Build history of the part. All positions in model axes, mm. Face numbers are marked on the shaded views. A direction names the side the tool comes from. Round coordinates to 2 decimals unless told otherwise and drop trailing zeros. Order: outer loops, then holes, each group sorted by start corner. A loop starts at its lowest first (then second) coordinate and runs counter-clockwise, first axis right, second up. Notation, with made-up numbers: M -28,19.5 L 5,19.5 A14 cw 5,36.5 Z; hole C 71,-7 d1. An arc over 180 degrees is marked long. One line per question, with ' | ' between items. Start each with the question number.
from build123d import *

# Parameters (mm, degrees)
SKETCH1_R           = 2.5
BOSS_EXTRUDE1_DEPTH = 10
SKETCH2_W           = 4
SKETCH2_H           = 61.321004691
CUT_EXTRUDE1_DEPTH  = 3
FILLET1_R           = 5
CHAMFER2_SIZE       = 4
CHAMFER3_SIZE       = 4
SKETCH3_R           = 2.5
CUT_EXTRUDE2_DEPTH  = 10


with BuildPart() as part:
    # Sketch1 → Boss-Extrude1 (new body)
    with BuildSketch(Plane(origin=(0, 0, 0), x_dir=(1, 0, 0), z_dir=(0, 1, 0))):
        Polygon((0, -25), (0, 25), (15, 25), (15, -8), (20, -16), (24.76, -16), (24.76, -22.47), (30.26, -22.47), (30.26, -18), (35, -18), (120, -18), (120, -33), (5, -33), align=None)
        with Locations(Location((5, 20, 0), (0, 0, 270))):
            Circle(SKETCH1_R, mode=Mode.SUBTRACT)
        with Locations(Location((5, -20, 0), (0, 0, 270))):
            Circle(SKETCH1_R, mode=Mode.SUBTRACT)
    extrude(amount=BOSS_EXTRUDE1_DEPTH)

    # Sketch2 → Cut-Extrude1 (cut)
    with BuildSketch(Plane(origin=(0, 10, 0), x_dir=(1, 0, 0), z_dir=(0, 1, 0))):
        with Locations((12, -5.660502345)):
            Rectangle(SKETCH2_W, SKETCH2_H)
    extrude(amount=-CUT_EXTRUDE1_DEPTH, mode=Mode.SUBTRACT)

    # Fillet1
    fillet1_edges = [part.edges().sort_by_distance(p)[0] for p in [
        (120, 5, 33),
        (120, 5, 18),
        (0, 5, -25),
        (15, 5, -25),
    ]]
    fillet(fillet1_edges, radius=FILLET1_R)

    # Chamfer2
    # the kernel refuses this chamfer: 4 mm, written as the material it takes off along each edge
    with BuildSketch(Plane(origin=(115, 10, 33), x_dir=(0, -0.9996219169112968, 0.02749587661058563), z_dir=(-1, 0, 0))) as chamfer2_piece_1:
        Polygon((CHAMFER2_SIZE * 0.999621916911, -CHAMFER2_SIZE * 0.0274958766106), (-CHAMFER2_SIZE * 0.0274958766106, -CHAMFER2_SIZE * 0.999621916911), (0, 0), align=None)
    extrude(amount=111.286731952, mode=Mode.SUBTRACT)
    with BuildSketch(Plane(origin=(20.286731952, 10, 33), x_dir=(0, 0.027495876610586487, -0.9996219169112968), z_dir=(-1, 0, 0))) as chamfer2_piece_2:
        Polygon((CHAMFER2_SIZE * 0.999621916911, CHAMFER2_SIZE * 0.0274958766106), (-CHAMFER2_SIZE * 0.0274958766106, CHAMFER2_SIZE * 0.999621916911), (0, 0), align=None)
    extrude(amount=25.573463904, mode=Mode.SUBTRACT)
    with BuildSketch(Plane(origin=(115, 10, 28), x_dir=(0, 0, 1), z_dir=(-1, 0, 0))) as chamfer2_piece_3:
        Polygon((5, -CHAMFER2_SIZE), (5 - CHAMFER2_SIZE, 0), (5, 0), align=None)
    revolve(axis=Axis((115, 10, 28), (0, 1, 0)), revolution_arc=90, mode=Mode.SUBTRACT)
    with BuildSketch(Plane(origin=(120, 10, 23), x_dir=(0.02749587661058563, -0.9996219169112968, 0), z_dir=(0, 0, 1))) as chamfer2_piece_4:
        Polygon((CHAMFER2_SIZE * 0.999621916911, -CHAMFER2_SIZE * 0.0274958766106), (-CHAMFER2_SIZE * 0.0274958766106, -CHAMFER2_SIZE * 0.999621916911), (0, 0), align=None)
    extrude(amount=5, mode=Mode.SUBTRACT)
    with BuildSketch(Plane(origin=(115, 10, 23), x_dir=(0, 0, -1), z_dir=(-1, 0, 0))) as chamfer2_piece_5:
        Polygon((5, CHAMFER2_SIZE), (5 - CHAMFER2_SIZE, 0), (5, 0), align=None)
    revolve(axis=Axis((115, 10, 23), (0, -1, 0)), revolution_arc=90, mode=Mode.SUBTRACT)
    with BuildSketch(Plane(origin=(30.26, 10, 18), x_dir=(0, -0.9996219169112968, -0.027495876610586494), z_dir=(1, 0, 0))) as chamfer2_piece_6:
        Polygon((CHAMFER2_SIZE * 0.999621916911, -CHAMFER2_SIZE * 0.0274958766106), (-CHAMFER2_SIZE * 0.0274958766106, -CHAMFER2_SIZE * 0.999621916911), (0, 0), align=None)
    extrude(amount=84.74, mode=Mode.SUBTRACT)

    # Chamfer3
    chamfer3_edges = [part.edges().sort_by_distance(p)[0] for p in [
        (22.38, 10, 16),
        (17.5, 10, 12),
    ]]
    chamfer(chamfer3_edges, length=CHAMFER3_SIZE)

    # Sketch3 → Cut-Extrude2 (cut)
    with BuildSketch(Plane(origin=(0, 10, 0), x_dir=(1, 0, 0), z_dir=(0, 1, 0))):
        with Locations(Location((27.5, -27, 0), (0, 0, 270))):
            Circle(SKETCH3_R)
    extrude(amount=-CUT_EXTRUDE2_DEPTH, mode=Mode.SUBTRACT)


solid = part.part
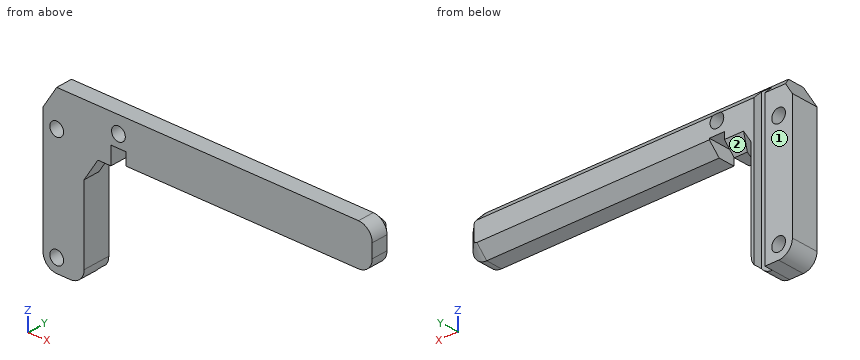
Item 1: Cut at B-B on x = 54. Write the cut outline in (y, z), then the cut area to 3 significant figures.
Item 2: Tool access for the marked faces 1 and 2: list every direction of +Z, -Z, +X, -X, +Y, -Y with a clear straight run to the whole face (end or side of a thin tool).
Item 3: Flat gauge pins, fed straight in: pin 1 (1.4 mm diameter, centred on x = 21.5, y = 4.5, fed in from -Z); pin 2 (4.5 mm diameter, centred on x = 5, z = 20, fed in from -Y); pin 3 (5 mm diameter, centred on x = 71.5, y = 2, fed in from -Z); pin 4 (2 mm diameter, centred on x = 12, z = 17, fed in from +Y). Where does each tip first touch, or does it go through?
Item 4: Cut at A-A on y = 4.25. Write the cut outline in (x, z), then the cut area to 3 significant figures.
Item 5: Wall check: line 1 along X through (y, z) = (7.5, -20); line 2 along Z through (x, y) = (27.5, 7); line 3 along Z through (x, y) = (6, 4). Give the ranges that are in metal, low to high. Write a range as [from, to].
Item 6: Cut at C-C on z = -4. Write the cut outline in (x, y).
Results found:
1) outline: M 0,18 L 6,18 L 10,22 L 10,29 L 6,33 L 0,33 Z | area: 134 mm^2
2) face 1: +Z, -Z, +X, -X, +Y | face 2: -Z, +X, +Y
3) pin 1: stops at z = 16 | pin 2: passes through | pin 3: stops at z = 18 | pin 4: stops at y = 7
4) outline: M 0,-20 A5 ccw 5,-25 L 10,-25 A5 ccw 15,-20 L 15,8 L 20,16 L 24.76,16 L 24.76,22.47 L 30.26,22.47 L 30.26,18 L 115,18 A5 ccw 120,23 L 120,28 A5 ccw 115,33 L 5,33 L 0,25 Z; hole C 5,-20 d5; hole C 5,20 d5; hole C 27.5,27 d5 | area: 2,360 mm^2
5) line 1: x = [0, 2.5], [7.5, 10], [14, 15] | line 2: z = [22.47, 24.5], [29.5, 32] | line 3: z = [-25, -22.29], [-17.71, 17.71], [22.29, 33]
6) outline: M 0,0 L 15,0 L 15,10 L 14,10 L 14,7 L 10,7 L 10,10 L 0,10 Z
